Can you work these out from the model? Positions are in its coordinate system, mm. Give positions to 0.01 mm unless a question says otherwise; leave off trailing zeros. Loops run counter-clockwise (first coordinate to the right, second up) from the corner with the lowest first, then second, coordinate; pieces in that order, holes last.
from build123d import *


# Not quite as in the source:
# - a fillet or chamfer that OpenCascade refuses, or shapes differently, is made with other operations: its cross-section is extruded or revolved along the edge and cut away or added


with BuildPart() as f1:
    # F0 (on Front) → F1 (revolve)
    with BuildSketch(Plane.XZ):
        with BuildLine():
            Line((-44.4924347103, 0), (0, 0))
            Line((0, 0), (0, 65.1155337691))
            Line((0, 65.1155337691), (-44.4924347103, 65.1155337691))
            Line((-44.4924347103, 65.1155337691), (-44.4924347103, 56.7583087614))
            ThreePointArc((-44.4924347103, 56.7583087614), (-37.9552003214, 50.2210743725), (-44.4924347103, 43.6838399837))
            Line((-44.4924347103, 43.6838399837), (-44.4924347103, 22.9257815758))
            ThreePointArc((-44.4924347103, 22.9257815758), (-37.9887534996, 16.4221003652), (-44.4924347103, 9.9184191545))
            Line((-44.4924347103, 9.9184191545), (-44.4924347103, 0))
        make_face()
    revolve(axis=Axis((0, 0, 32.5577668846), (0, 0, 1)))

    # F2: chamfer of 5.08 on 4 edges, made by hand

    # F2_s1 → F2_t2 (revolve, cut)
    with BuildSketch(Plane.XZ):
        Polygon((-39.4124347103, 65.1155337691), (-44.4924347103, 60.0355337691), (-44.4924347103, 65.1155337691), align=None)
    revolve(axis=Axis((0, 0, 65.1155337691), (0, 0, 1)), mode=Mode.SUBTRACT)

    # F2_s3 → F2_t4 (revolve, cut)
    with BuildSketch(Plane.XZ):
        with BuildLine():
            Line((-44.4924347103, 6.0117559717), (-41.6402584505, 10.5771914803))
            ThreePointArc((-41.6402584505, 10.5771914803), (-42.9562364784, 10.1024513019), (-44.4924347103, 9.9184191545))
            Line((-44.4924347103, 9.9184191545), (-44.4924347103, 6.0117559717))
        make_face()
    revolve(axis=Axis((0, 0, 9.9184191545), (0, 0, 1)), mode=Mode.SUBTRACT)

    # F2_s5 → F2_t6 (revolve, cut)
    with BuildSketch(Plane.XZ):
        Polygon((-44.4924347103, 5.08), (-39.4124347103, 0), (-44.4924347103, 0), align=None)
    revolve(axis=Axis((0, 0, 0), (0, 0, 1)), mode=Mode.SUBTRACT)


solid = f1.part
(1) Suppose I cut it at A-A on x = 0. List the corners of the cut face in (y, z) for me.
Returned:
outline: (-44.49, 5.08) - (-39.41, 0) - (39.41, 0) - (44.49, 5.08) - (44.49, 6.01) - (41.64, 10.58) arc R6.5 cw to (44.49, 22.93) - (44.49, 43.68) arc R6.54 cw to (44.49, 56.76) - (44.49, 60.04) - (39.41, 65.12) - (-39.41, 65.12) - (-44.49, 60.04) - (-44.49, 56.76) arc R6.54 cw to (-44.49, 43.68) - (-44.49, 22.93) arc R6.5 cw to (-41.64, 10.58) - (-44.49, 6.01) - close
(2) Will these pins go through, and if not, where does the flat tip stop? P1, Ø1, axis at y = 7, z = 23.5, coming from the -X side; P2, Ø1, axis at y = -34.5, z = 8, coming from the -X side; P3, Ø1, axis at x = -13.5, z = 40, coming from the +Y side.
Returned:
P1: stops at x = -44.02
P2: stops at x = -26.91
P3: stops at y = 42.55
(3) Suppose I cut it at C-C on z = 42.5. List the corners of the cut face in (x, y) for me.
Returned:
outline: circle Ø88.98 at (0, 0)
(4) Thinking about a two-plate mould opening in Z: for faces 1 (the conical face through (9.057, 40.785, 10.356)), 2 (the cylindrical face through (-42.44, -13.36, 58.37)), 3 (the flat face through (1, -1, 0)), which applies, pulls with the +Z half, pulls with the -Z half, needs draft (parallel to the pull), parting line crosses it, or undercut?
Returned:
face 1: undercut
face 2: needs draft
face 3: pulls with the -Z half
(5) Please list where these lines run through material, in increasing order: probe 1 along Z at (x, y) = (-14, -40); probe 2 along Z at (x, y) = (34, 19.5); probe 3 along Y at (x, z) = (5, 33.5).
Returned:
probe 1: z = 2.97 to 9.39, 22.57 to 44.03, 56.41 to 62.15
probe 2: z = 0 to 12.65, 20.2 to 46.39, 54.05 to 65.12
probe 3: y = -44.21 to 44.21
